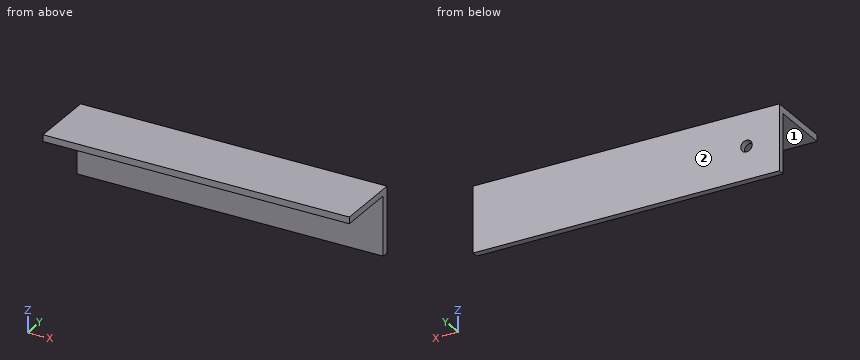
from build123d import *

# Parameters (mm, degrees)
PAD_DEPTH            = 372.752246
SKETCH001_R          = 7
POCKET_DEPTH         = 80.001
BODY_ROLL_ANGLE      = -90
BODY_PLACEMENT_ANGLE = 180


with BuildPart() as part:
    # Sketch → Pad (new body)
    with BuildSketch(Plane.YZ):
        Polygon((0, 0), (0, 80), (8, 80), (8, 8), (80, 8), (80, 0), align=None)
    extrude(amount=PAD_DEPTH)

    # Sketch001 (on Face6 of Pad) → Pocket (cut, through all)
    with BuildSketch(Plane.YX):
        with Locations((40, 332.752246)):
            Circle(SKETCH001_R)
    extrude(amount=-POCKET_DEPTH, mode=Mode.SUBTRACT)


with BuildPart() as part_1:
    # Body roll: moved
    add(part.part.rotate(Axis((0, 0, 0), (1, 0, 0)), BODY_ROLL_ANGLE))


with BuildPart() as part_2:
    # Body placement: moved
    add(part_1.part.moved(Location((-80, 80, 0))).rotate(Axis((-80, 80, 0), (0, 0, 1)), BODY_PLACEMENT_ANGLE))


solid = part_2.part
The model under review builds one solid part; all positions refer to its coordinate system, in mm. Face numbers are marked on the shaded views. A direction names the side the tool comes from. Round coordinates to 2 decimals unless told otherwise and drop trailing zeros. Loops run counter-clockwise (first coordinate to the right, second up) from the corner with the lowest first, then second, coordinate; pieces in that order, holes last. Notation, with made-up numbers: (-40, 13) - (19, 13) arc R19 ccw to (19, 30) - close; hole circle Ø7 at (29.25, -14). An arc over 180 degrees is marked (long way). Use CSV: the item, a comma, the result in double quotes.
(1) Take a section at B-B, the plane x = -298. Give the boundary of the cut face in (y, z).
Working result:
outline,"(0, -8) - (72, -8) - (72, -80) - (80, -80) - (80, 0) - (0, 0) - close"
(2) Take a section at C-C, the plane y = 53. Give the boundary of the cut face in (x, z), plus the area to 3 significant figures.
Working result:
outline,"(-452.75, -8) - (-80, -8) - (-80, 0) - (-452.75, 0) - close"
area,"2,980 mm^2"
(3) Machinability: for the marked faces 1 and 2, which of the approach directions +Z, -Z, +X, -X, +Y, -Y give a long, thin tool a straight path to every point of the face, cutting with its end or side? Answer none if there is none.
Working result:
face 1,"-Z, +X, -X, -Y"
face 2,"+Z, -Z, +X, -X, +Y"
(4) Clearance check with a flat-ended pin moving along its axis: P1, Ø2, axis at x = -151.5, y = 52.5, coming from the -Z side. State where the tip first meets the part, or that it passes through.
Working result:
P1,"stops at z = -8"
(5) For line 1 (X direction, y = 74.5, z = -40); line 2 (Z direction, x = -406, y = 24); line 3 (Y direction, x = -365, z = -22.5), list the stretches that pass through material, from the lowest coordinate up.
Working result:
line 1,"x = -452.75 to -419.75, -405.75 to -80"
line 2,"z = -8 to 0"
line 3,"y = 72 to 80"
(6) Take a section at A-A, the plane z = -40. Give the boundary of the cut face in (x, y), plus the area to 3 significant figures.
Working result:
outline,"(-452.75, 72) - (-419.75, 72) - (-419.75, 80) - (-452.75, 80) - close; (-405.75, 72) - (-80, 72) - (-80, 80) - (-405.75, 80) - close"
area,"2,870 mm^2"
